Input: part model. Units: mm. Frame: model coordinates. Face numbers are marked on the shaded views. A direction names the side the tool comes from. Coordinates: 2 decimals unless noted, no trailing zeros. Loops run counter-clockwise (first coordinate to the right, second up) from the corner with the lowest first, then second, coordinate; pieces in that order, holes last.
Solid Edge part; units mm, degrees
sketch "Sketch1" plane through (0, 0, 0) normal (0, 0, 1) x (1, 0, 0)
  line L0 (-120.65, -139.7) -> (120.65, -139.7)
  line L1 (120.65, -139.7) -> (120.65, 139.7)
  line L2 (120.65, 139.7) -> (-120.65, 139.7)
  line L3 (-120.65, 139.7) -> (-120.65, -139.7)
extrude "Protrusion1" add sketch "Sketch1" along normal mid plane 244.475
sketch "Sketch2" plane through (0, -139.7, 0) normal (0, -1, 0) x (1, 0, 0)
  line L0 (-120.65, 122.2375) -> (120.65, 122.2375)
  line L1 (120.65, 122.2375) -> (120.65, 68.2625)
  line L2 (120.65, 68.2625) -> (-120.65, 68.2625)
  line L3 (-120.65, 68.2625) -> (-120.65, 122.2375)
extrude "Cutout1" cut sketch "Sketch2" against normal up to vertex (279.4 mm away)
shell "Thinwall_1" thickness 38.1 removed faces 1 at (82.8463, 90.3393, 68.2625)
fillet "Round_1" radius 12.7 8 edges at (120.65, 139.7, -26.9875) (120.65, -139.7, -26.9875) (-120.65, -139.7, -26.9875) (-120.65, 139.7, -26.9875) (0, -139.7, -122.2375) (-120.65, 0, -122.2375) (120.65, 0, -122.2375) (0, 139.7, -122.2375)
fillet "Round_2" radius 6.35 4 edges at (-82.55, 101.6, -7.9375) (82.55, 101.6, -7.9375) (82.55, -101.6, -7.9375) (-82.55, -101.6, -7.9375)
sketch "Sketch3" plane through (120.65, 0, -96.8375) normal (1, 0, 0) x (0, 1, 0)
  circle A0 centre (-88.9, 139.7) radius 3.5
  circle A1 centre (88.9, 139.7) radius 3.5
  circle A2 centre (88.9, 0) radius 3.5
  circle A3 centre (-88.9, 0) radius 3.5
extrude "ExtrudedCutout_2" cut sketch "Sketch3" against normal blind 25.4
chamfer "Chamfer_1" distance 6.35 angle 22.5 1 edges at (120.65, -92.4, 42.8625) measured on face at (99.7373, -86.9631, 45.7777)
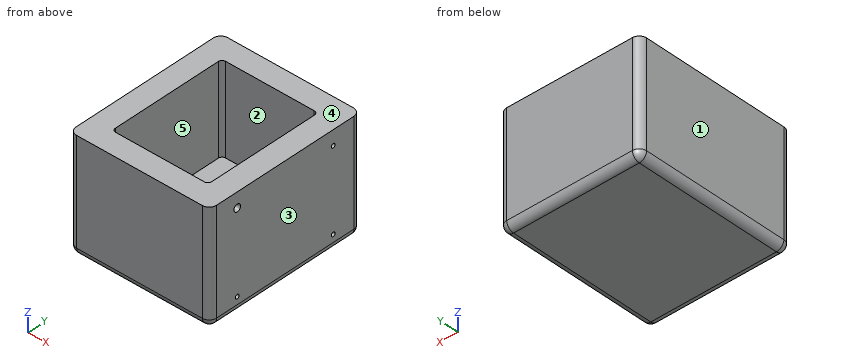
Item 1: Mould query, pull axis X, two halves, no side actions, for the marked faces 3, 4 and 5. Classes: +X half, -X half, draft (parallel to the pull), parting line (faces both ways), or undercut.
Result:
face 3: +X half
face 4: draft
face 5: undercut
Item 2: Section query B-B (y = 74). Output: boundary loops of the cut face in (x, z), then the cut area to 3 significant figures.
Result:
outline: (-120.65, -109.54) arc R12.7 ccw to (-107.95, -122.24) - (107.95, -122.24) arc R12.7 ccw to (120.65, -109.54) - (120.65, 68.26) - (82.55, 68.26) - (82.55, -84.14) - (-82.55, -84.14) - (-82.55, 68.26) - (-120.65, 68.26) - close
area: 20,700 mm2
Item 3: Contact query for flat-ended pins moving along their axis: P1, Ø5.5, axis at y = -89, z = 41.5, coming from the +X side; P2, Ø6.5, axis at y = 88.9, z = -96.84, coming from the +X side; P3, Ø5, axis at x = -56, y = 97.5, coming from the +Z side. Output: stop coordinate, or through.
Result:
P1: stops at x = 115.79
P2: stops at x = 95.25
P3: stops at z = -84.14
Item 4: Section query C-C (x = 1). Output: boundary loops of the cut face in (y, z), then the cut area to 3 significant figures.
Result:
outline: (-139.7, -109.54) arc R12.7 ccw to (-127, -122.24) - (127, -122.24) arc R12.7 ccw to (139.7, -109.54) - (139.7, 68.26) - (101.6, 68.26) - (101.6, -84.14) - (-101.6, -84.14) - (-101.6, 68.26) - (-139.7, 68.26) - close
area: 22,200 mm2
Item 5: Reachability of the marked faces 1 and 2 from +Z, -Z, +X, -X, +Y, -Y: full face, straight path, thin tool, end or side. Return the list, or none.
Result:
face 1: +Z, -Z, -X, +Y, -Y
face 2: +Z
Item 6: Line query: L1, parallel to Y at x = -64.5, z = 6; L2, parallel to X at y = -41, z = 14.5; L3, parallel to Z at x = 101, y = 88. Output: solid intervals per line, ascending.
Result:
L1: y = -139.7 to -101.6, 101.6 to 139.7
L2: x = -120.65 to -82.55, 82.55 to 120.65
L3: z = -122.24 to -100.22, -93.46 to 39.48, 46.24 to 68.26
Item 7: Section query A-A (z = -22). Output: boundary loops of the cut face in (x, y), then the cut area to 3 significant figures.
Result:
outline: (-120.65, -127) arc R12.7 ccw to (-107.95, -139.7) - (107.95, -139.7) arc R12.7 ccw to (120.65, -127) - (120.65, 127) arc R12.7 ccw to (107.95, 139.7) - (-107.95, 139.7) arc R12.7 ccw to (-120.65, 127) - close; hole (-82.55, -95.25) arc R6.35 ccw to (-76.2, -101.6) - (76.2, -101.6) arc R6.35 ccw to (82.55, -95.25) - (82.55, 95.25) arc R6.35 ccw to (76.2, 101.6) - (-76.2, 101.6) arc R6.35 ccw to (-82.55, 95.25) - close
area: 33,800 mm2
Item 8: Section query D-D (y = -88.9). Output: boundary loops of the cut face in (x, z), then the cut area to 3 significant figures.
Result:
outline: (-120.65, -109.54) arc R12.7 ccw to (-107.95, -122.24) - (107.95, -122.24) arc R12.7 ccw to (120.65, -109.54) - (120.65, -100.34) - (95.25, -100.34) - (95.25, -93.34) - (120.65, -93.34) - (120.65, 36.73) - (114.3, 39.36) - (95.25, 39.36) - (95.25, 46.36) - (114.3, 46.36) - (120.65, 48.99) - (120.65, 68.26) - (82.55, 68.26) - (82.55, -84.14) - (-82.55, -84.14) - (-82.55, 68.26) - (-120.65, 68.26) - close
area: 20,400 mm2
